For this review, take the finished solid that the model builds, in its own axes (mm). A direction names the side the tool comes from. Give positions to 0.01 mm unless a question says otherwise; leave off trailing zeros. Order: outer loops, then holes, each group sorted by start corner. A loop starts at its lowest first (then second) coordinate and runs counter-clockwise, first axis right, second up.
Autodesk Inventor part; units mm, degrees
ref_plane "YZ Plane" through (0, 0, 0) normal (1, 0, 0) x (0, 1, 0)
ref_plane "XZ Plane" through (0, 0, 0) normal (0, 1, 0) x (-1, 0, 0)
ref_plane "XY Plane" through (0, 0, 0) normal (0, 0, 1) x (1, 0, 0)
sketch "Sketch1" plane through (0, 0, 0) normal (0, 0, 1) x (1, 0, 0)
  line L0 (-70, -115) -> (70, -115)
  line L1 (70, -115) -> (70, 115)
  line L2 (70, 115) -> (-70, 115)
  line L3 (-70, 115) -> (-70, -115)
  point P0 (0, 0)
  dimension "width" = 140
  dimension "d1" = 70
  dimension "d2" = 230
  dimension "d3" = 115
extrude "Extrusion1" add sketch "Sketch1" along normal blind 5
sketch "Sketch2" plane through (0, 0, 5) normal (0, 0, 1) x (1, 0, 0)
  circle A0 centre (-45, 69) radius 15.5
  circle A1 centre (-15, 93) radius 15.5
  point P0 (0, 0)
  dimension "d6" = 31
  dimension "d7" = 69
  dimension "d8" = 45
  dimension "d17" = 31
  dimension "d18" = 30
  dimension "d19" = 24
extrude "Extrusion2" cut sketch "Sketch2" against normal blind 5
pattern_linear "Rectangular Pattern2" count 2 spacing 60 along (1, 0, 0) count 4 spacing 48 along (0, -1, 0) of "Extrusion2"
sketch "Sketch3" plane through (0, 0, 5) normal (0, 0, 1) x (1, 0, 0)
  line L0 (-70, -115) -> (70, -115)
  line L1 (-70, -115) -> (-45, -115)
  line L2 (-45, -115) -> (-45, -110)
  line L3 (-45, -110) -> (-70, -110)
  line L4 (-70, -110) -> (-70, -115)
  line L5 (-70, 115) -> (-70, -115)
  line L6 (-70, 115) -> (-60, 115)
  line L7 (-60, 115) -> (-60, 110)
  line L8 (-60, 110) -> (-70, 110)
  line L9 (-70, 110) -> (-70, 115)
  line L10 (-70, -115) -> (-65, -115)
  line L11 (-65, -115) -> (-65, -90)
  line L12 (-65, -90) -> (-70, -90)
  line L13 (-70, -90) -> (-70, -115)
  line L14 (-70, 115) -> (-65, 115)
  line L15 (-65, 115) -> (-65, 90)
  line L16 (-65, 90) -> (-70, 90)
  line L17 (-70, 90) -> (-70, 115)
  point P0 (0, 0)
  dimension "d26" = 5
  dimension "d27" = 25
  dimension "d28" = 5
  dimension "d29" = 10
  dimension "d30" = 5
  dimension "d31" = 25
  dimension "d32" = 5
  dimension "d33" = 25
extrude "Extrusion3" cut sketch "Sketch3" against normal blind 10
mirror "Mirror1" about plane through (0, 0, 0) normal (1, 0, 0) of "Extrusion3"
sketch "Sketch4" plane through (0, 0, 5) normal (0, 0, 1) x (1, 0, 0)
  line L0 (-45, -115) -> (45, -115)
  line L1 (-25, -115) -> (25, -115)
  line L2 (25, -115) -> (25, -100)
  line L3 (25, -100) -> (-25, -100)
  line L4 (-25, -100) -> (-25, -115)
  point P0 (0, 0)
  dimension "d36" = 25
  dimension "d37" = 50
  dimension "d38" = 15
extrude "Extrusion4" cut sketch "Sketch4" against normal blind 10
fillet "Fillet1" radius 5 2 edges at (-25, -100, 2.5) (25, -100, 2.5)
equation "\"d17\" = d6"
equation "\"d22\" = 2 * d18"
equation "\"d25\" = 2 * d19"
equation "\"d30\" = d26"
equation "\"d31\" = d27"
equation "\"d32\" = d28"
properties part number "EBF_001.1-top-plate_cup-holder"
1) Tool access review of faces 1 (the face through (-24, -102, 2)), 2 (the face through (65, -100, 3)), 3 (the face through (-65, 100, 3)), 4 (the face through (-67, -90, 3)), 5 (the face through (68, 90, 3)): name each direction out of +Z, -Z, +X, -X, +Y, -Y from which nothing blocks a thin tool from reaching the whole face with its end or side.
Answer sheet:
face 1: +Z, -Z, -Y
face 2: +Z, -Z, +X, -Y
face 3: +Z, -Z, -X, +Y
face 4: +Z, -Z, -X, -Y
face 5: +Z, -Z, +X, +Y
2) We need section B-B on x = -15. Give the boundary of the cut face in (y, z), then the cut area to 3 significant figures.
Answer sheet:
outline: (-100, 0) - (-66.5, 0) - (-66.5, 5) - (-100, 5) - close; (-35.5, 0) - (-18.5, 0) - (-18.5, 5) - (-35.5, 5) - close; (12.5, 0) - (29.5, 0) - (29.5, 5) - (12.5, 5) - close; (60.5, 0) - (77.5, 0) - (77.5, 5) - (60.5, 5) - close; (108.5, 0) - (115, 0) - (115, 5) - (108.5, 5) - close
area: 455 mm2
3) Clearance check with flat-ended pins moving along their axes: pin 1 (1.5 mm diameter, centred on x = -68.5, z = 2, fed in from -Y); pin 2 (2.5 mm diameter, centred on x = 63, z = 1.5, fed in from +Y); pin 3 (2.5 mm diameter, centred on y = -109.5, z = 3, fed in from +X); pin 4 (5 mm diameter, centred on x = 28, y = 67, fed in from +Z). State where each tip first meets the part, or that it passes through.
Answer sheet:
pin 1: stops at y = -90
pin 2: stops at y = 110
pin 3: stops at x = 65
pin 4: stops at z = 5
4) We need section A-A on y = -27. Give the boundary of the cut face in (x, z).
Answer sheet:
outline: (-70, 0) - (-60.5, 0) - (-60.5, 5) - (-70, 5) - close; (-29.5, 0) - (-0.5, 0) - (-0.5, 5) - (-29.5, 5) - close; (30.5, 0) - (70, 0) - (70, 5) - (30.5, 5) - close
5) Draft analysis for pull direction X (two halves, no side actions). For faces 6 (the face through (-30.485, -2.318, 2.535)), 7 (the face through (-60, 113, 3)), 8 (the face through (45, -112, 3)), 9 (the face through (1, 115, 2)), state which applies: +X half, -X half, draft (parallel to the pull), parting line (faces both ways), or undercut.
Answer sheet:
face 6: undercut
face 7: -X half
face 8: +X half
face 9: draft
6) We need section C-C on z = 3.75. Count the separate pieces of the cut face and the enclosed holes in it, then the cut area to 3 significant figures.
Answer sheet:
separate pieces: 1
enclosed holes: 16
area: 18,600 mm2
7) We need section D-D on x = 36. Give the boundary of the cut face in (y, z), then the cut area to 3 significant figures.
Answer sheet:
outline: (-115, 0) - (-63.62, 0) - (-63.62, 5) - (-115, 5) - close; (-38.38, 0) - (-15.62, 0) - (-15.62, 5) - (-38.38, 5) - close; (9.62, 0) - (32.38, 0) - (32.38, 5) - (9.62, 5) - close; (57.62, 0) - (80.38, 0) - (80.38, 5) - (57.62, 5) - close; (105.62, 0) - (115, 0) - (115, 5) - (105.62, 5) - close
area: 645 mm2
8) To check wall thickness, follow line 1 (Y direction, x = 15, z = 3.35); line 2 (X direction, y = -26, z = 4.8); line 3 (Y direction, x = -52, z = 0.85). State the ranges of each line that lie inside material, in increasing order.
Answer sheet:
line 1: y = -100 to -90.5, -59.5 to -42.5, -11.5 to 5.5, 36.5 to 53.5, 84.5 to 115
line 2: x = -70 to -60.47, -29.53 to -0.47, 30.47 to 70
line 3: y = -110 to -88.83, -61.17 to -40.83, -13.17 to 7.17, 34.83 to 55.17, 82.83 to 115
